Model file for the job. Use its own axes, mm. A direction names the side the tool comes from. Coordinates: 2 decimals unless noted, no trailing zeros. Loops run counter-clockwise (first coordinate to the right, second up) from the corner with the lowest first, then second, coordinate; pieces in that order, holes last.
Autodesk Fusion 360 part; units mm, degrees
sketch "Esquisse1" plane through (0, 0, 0) normal (0, 0, 1) x (1, 0, 0)
  circle A0 centre (0, 0) radius 3.5
  circle A1 centre (0, 0) radius 6
  line L0 (1.8028, -3) -> (-1.8028, -3)
  line L1 (-1.8028, -3) -> (-1.8028, -3.5)
  line L2 (-1.8028, -3.5) -> (1.8028, -3.5)
  line L3 (1.8028, -3.5) -> (1.8028, -3)
  dimension "d1" = 7
  dimension "d2" = 12
  dimension "d17" = 0.5
extrude "Extrusion1" add sketch "Esquisse1" along normal blind 15 contours A0 L0 | A0 L1 L2 | A0 L2 L3 | A1 picked at (0.4606, -3.0719)
ref_plane "Plan de construction1" through (0, 0, 20) normal (0, 0, 1) x (1, 0, 0)
sketch "Esquisse2" plane through (0, 0, 20) normal (0, 0, 1) x (1, 0, 0)
  line L0 (-1.8708, 1.25) -> (1.8708, 1.25)
  line L1 (1.8708, -1.25) -> (-1.8708, -1.25)
  arc A0 (-1.8708, 1.25) -> (-1.8708, -1.25) centre (0, 0) ccw
  arc A1 (1.8708, -1.25) -> (1.8708, 1.25) centre (0, 0) ccw
  dimension "d6" = 4.5
  dimension "d16" = 2.5
sketch "Esquisse3" plane through (0, 0, 15) normal (0, 0, 1) x (1, 0, 0)
  circle A0 centre (0, 0) radius 6
  circle A1 centre (0, 0) radius 6
  arc A2 (1.8028, -3) -> (-1.8028, -3) centre (0, 0) ccw
  line L0 (1.8028, -3) -> (-1.8028, -3)
  dimension "d13" = 12
loft "Lissage1" add profiles "Esquisse3", "Esquisse2" section 1 contours A0 A1 | A2 L0 section 2
extrude "Extrusion2" add 1 faces at (0.6236, -0.4167, 20) along direction (0, 0, 1) blind 25
sketch "Esquisse4" plane through (0, 0, 0) normal (0, 1, 0) x (1, 0, 0)
  circle A0 centre (0, -5) radius 1.5
  line L0 (0, 0) -> (0, -15) construction
  line L1 (-4.9889, -15) -> (4.9889, -15)
  dimension "d11" = 3
  dimension "d12" = 5
extrude "Extrusion3" cut sketch "Esquisse4" against normal blind 10
equation "d9 = 5 mm + 3 mm + 5 mm + 5 mm + 7 mm"
Q1. Slice it at C-C (z = 5). List the corners of the cut face in (x, y).
Answers:
outline: (-1.8, -3) arc R3.5 cw (long way) to (1.8, -3) - (1.5, -3) - (1.5, -5.81) arc R6 ccw (long way) to (-1.5, -5.81) - (-1.5, -3) - close
Q2. Slice it at B-B (z = 40). List the corners of the cut face in (x, y), and give its area (3 significant figures).
Answers:
outline: (-1.87, -1.25) - (1.87, -1.25) arc R2.25 ccw to (1.87, 1.25) - (-1.87, 1.25) arc R2.25 ccw to start
area: 10.6 mm2
Q3. Flat gauge pins, fed straight in: P1, Ø4, axis at x = 0.5, z = 35, coming from the -Y side; P2, Ø1.1, axis at x = 0.5, z = 34, coming from the +Y side; P3, Ø3, axis at x = -4, y = 2, coming from the +Z side. Where does each tip first touch, or does it go through?
Answers:
P1: stops at y = -1.25
P2: stops at y = 1.25
P3: stops at z = 19.04
Q4. Drill centre lines: line 1 (X direction, y = 0, z = 8.5); line 2 (Y direction, x = 0, z = 10.5); line 3 (Y direction, x = 0, z = 6). Where is each one in solid material? Low to high.
Answers:
line 1: x = -6 to -3.5, 3.5 to 6
line 2: y = -6 to -3, 3.5 to 6
line 3: y = 3.5 to 6
Q5. Slice it at A-A (y = 0). List the corners of the cut face in (x, z).
Answers:
outline: (-6, 0) - (-3.5, 0) - (-3.5, 15) - (3.5, 15) - (3.5, 0) - (6, 0) - (6, 15) - (2.25, 20) - (2.25, 45) - (-2.25, 45) - (-2.25, 20) - (-6, 15) - close
Q6. Which spindle directions (+Z, -Z, +X, -X, +Y, -Y) get a long thin tool onto all of the face, cutting with end or side? Do faces 4 (the cylindrical face through (2.25, 0.02, 32.33)), 5 (the cylindrical face through (1.43, -4.48, 4.55)), 6 (the cylindrical face through (-2.25, -0.02, 32.33)), 7 (the flat face through (0, 1.25, 32)). Say none if no direction does.
Answers:
face 4: +Z, +X
face 5: -Y
face 6: +Z, -X
face 7: +Z, +X, -X, +Y
Q7. Mould opens along X. For faces 1 (the flat face through (0, 0, 45)), 2 (the conical face through (-4.151, -0.034, 17.465)), 3 (the flat face through (0, 0, 15)) say: +X half, -X half, draft (parallel to the pull), parting line (faces both ways), or undercut.
Answers:
face 1: draft
face 2: -X half
face 3: undercut
